Verification items for the finished model (mm, model axes). Give positions to 0.01 mm unless a question says otherwise; leave off trailing zeros. Loops run counter-clockwise (first coordinate to the right, second up) from the corner with the lowest first, then second, coordinate; pieces in that order, holes last. Notation, with made-up numbers: (26.25, 74.25) - (69.25, 74.25) arc R33 cw to (69.25, 105.25) - close; hole circle Ø9 at (84, 70). An arc over 180 degrees is marked (long way). Put each result on its own line as item: value. Start each with the question number.
Autodesk Inventor part; units mm, degrees
ref_plane "Work Plane1" through (4, 0, 0) normal (1, 0, 0) x (0, 1, 0)
ref_plane "XZ Plane" through (0, 0, 0) normal (0, 1, 0) x (-1, 0, 0)
ref_plane "XY Plane" through (0, 0, 0) normal (0, 0, 1) x (1, 0, 0)
sketch "Sketch1" plane through (0, 0, 0) normal (0, 0, 1) x (1, 0, 0)
  circle A0 centre (0, 0) radius 4
  dimension "d0" = 8
extrude "Extrusion1" add sketch "Sketch1" along normal blind 96
ref_plane "Work Plane1" through (4, 0, 0) normal (1, 0, 0) x (0, 1, 0)
sketch "Sketch2" plane through (4, 0, 0) normal (1, 0, 0) x (0, 1, 0)
  point P0 (0, 0)
  point P1 (0, 2.5)
  dimension "d4" = 2.5
hole "Hole1" at (4, 0, 2.5) direction (-1, 0, 0) diameter 3 end through all
chamfer "Chamfer1" distance 0.5 angle 45 1 edges at (-4, 0, 96)
properties part number "201 part 5" material "Aluminum 6061-AHC"
1) Draft check along Z on faces 1 (the face through (0, 0, 0)), 2 (the face through (0, 0, 96)), 3 (the face through (-0.1, 0.9, 3.7)). Enter one of: pulls with the +Z half, pulls with the -Z half, needs draft (parallel to the pull), parting line crosses it, or undercut.
2) Section check A-A, the plane y = 0. Enter the section's corners in (x, z), plus the area to 3 significant figures.
3) Scan lines: line 1 along Z through (x, y) = (-2, 0); line 2 along Y through (x, z) = (0, 2.5); line 3 along Z through (x, y) = (-1, 0.75). Record each from-to range of solid material in increasing order. Write a range as from..to.
4) Section check C-C, the plane z = 15. Enter the section's corners in (x, y).
5) Depth check by flat-ended pin: P1, Ø4, axis at y = 3, z = 81.5, coming from the -X side. Enter the tip coordinate at first touch or a pass-through.
6) Section check B-B, the plane z = 2.5. Enter the section's corners in (x, y), plus the area to 3 significant figures.
Results are:
1. face 1: pulls with the -Z half
1. face 2: pulls with the +Z half
1. face 3: undercut
2. outline: (-4, 0) - (4, 0) - (4, 1) - (-4, 1) - close; (-4, 4) - (4, 4) - (4, 95.5) - (3.5, 96) - (-3.5, 96) - (-4, 95.5) - close
2. area: 744 mm2
3. line 1: z = 0..1, 4..96
3. line 2: y = -4..-1.5, 1.5..4
3. line 3: z = 0..1.2, 3.8..96
4. outline: circle Ø8 at (0, 0)
5. P1: stops at x = -3.87
6. outline: (-3.71, -1.5) arc R4 ccw to (3.71, -1.5) - close; (-3.71, 1.5) - (3.71, 1.5) arc R4 ccw to start
6. area: 26.8 mm2
